```python
from build123d import *

# Parameters (mm, degrees)
SKETCH1_W           = 20
SKETCH1_H           = 8
BOSS_EXTRUDE1_DEPTH = 20
SKETCH2_R           = 0.5
SKETCH2_R_2         = 1
SKETCH2_R_3         = 1.5
SKETCH2_R_4         = 2
CUT_EXTRUDE1_DEPTH  = 21


with BuildPart() as part:
    # Sketch1 → Boss-Extrude1 (new body)
    with BuildSketch(Plane.XY):
        with Locations((10, 4)):
            Rectangle(SKETCH1_W, SKETCH1_H)
    extrude(amount=-BOSS_EXTRUDE1_DEPTH)

    # Sketch2 → Cut-Extrude1 (cut, through all)
    with BuildSketch(Plane.XY):
        with Locations((4, 4)):
            Circle(SKETCH2_R)
        with Locations((7, 4)):
            Circle(SKETCH2_R_2)
        with Locations((11, 4)):
            Circle(SKETCH2_R_3)
        with Locations((16, 4)):
            Circle(SKETCH2_R_4)
    extrude(amount=-CUT_EXTRUDE1_DEPTH, mode=Mode.SUBTRACT)


solid = part.part
```
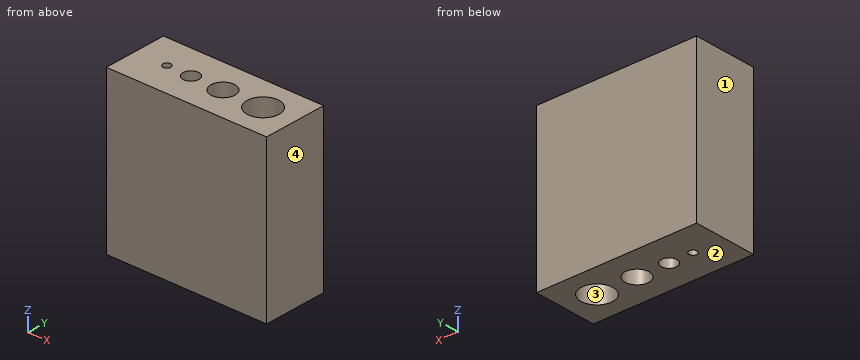
Can you work these out from the model? Positions are in its coordinate system, mm. Face numbers are marked on the shaded views. Round coordinates to 2 decimals unless told otherwise and drop trailing zeros. Loops run counter-clockwise (first coordinate to the right, second up) from the corner with the lowest first, then second, coordinate; pieces in that order, holes last. Notation, with made-up numbers: (36, -35.75) -> (64, -35.75) arc R33 ccw to (64, 2.25) -> close; hole circle Ø10 at (-22.5, -39.5). An arc over 180 degrees is marked (long way). One line per item, written item: value. Start each with the question number.
1. If we mould it in two halves opening along X, with no side actions, what happens to the marked faces 1, 2, 3 and 4? For each: pulls with the +X half, pulls with the -X half, needs draft (parallel to the pull), parting line crosses it, or undercut.
2. If we section it at A-A, the plane x = 16: Write out the boundary of the cut face in (y, z), then the cut area to 3 significant figures.
3. If we section it at C-C, the plane y = 4: Write out the boundary of the cut face in (x, z), then the cut area to 3 significant figures.
4. If I drill on probe 1 along Y at (x, z) = (4, -4.5); probe 2 along Y at (x, z) = (7, -4.75); probe 3 along X at (y, z) = (3.75, -16.75), over which ranges is the centre line in solid material (lowest first)?
5. If we section it at D-D, the plane y = 5.25: Write out the boundary of the cut face in (x, z), then the cut area to 3 significant figures.
6. If we section it at B-B, the plane z = -10.5: Write out the boundary of the cut face in (x, y), then the cut area to 3 significant figures.
Calculated:
1. face 1: pulls with the -X half
1. face 2: needs draft
1. face 3: undercut
1. face 4: pulls with the +X half
2. outline: (0, -20) -> (2, -20) -> (2, 0) -> (0, 0) -> close; (6, -20) -> (8, -20) -> (8, 0) -> (6, 0) -> close
2. area: 80.0 mm²
3. outline: (0, -20) -> (3.5, -20) -> (3.5, 0) -> (0, 0) -> close; (4.5, -20) -> (6, -20) -> (6, 0) -> (4.5, 0) -> close; (8, -20) -> (9.5, -20) -> (9.5, 0) -> (8, 0) -> close; (12.5, -20) -> (14, -20) -> (14, 0) -> (12.5, 0) -> close; (18, -20) -> (20, -20) -> (20, 0) -> (18, 0) -> close
3. area: 200 mm²
4. probe 1: y = 0 to 3.5, 4.5 to 8
4. probe 2: y = 0 to 3, 5 to 8
4. probe 3: x = 0 to 3.57, 4.43 to 6.03, 7.97 to 9.52, 12.48 to 14.02, 17.98 to 20
5. outline: (0, -20) -> (10.17, -20) -> (10.17, 0) -> (0, 0) -> close; (11.83, -20) -> (14.44, -20) -> (14.44, 0) -> (11.83, 0) -> close; (17.56, -20) -> (20, -20) -> (20, 0) -> (17.56, 0) -> close
5. area: 304 mm²
6. outline: (0, 0) -> (20, 0) -> (20, 8) -> (0, 8) -> close; hole circle Ø1 at (4, 4); hole circle Ø2 at (7, 4); hole circle Ø3 at (11, 4); hole circle Ø4 at (16, 4)
6. area: 136 mm²
